Here's how the part is built. I have some questions about the finished solid (model axes, mm). A direction names the side the tool comes from. Give positions to 0.01 mm unless a question says otherwise; leave off trailing zeros. Write each loop counter-clockwise with the first axis right and the second up, starting at its lowest first coordinate (ties: lowest second). Pieces come first, ordered by that corner, then holes. Notation, with made-up numbers: (-32.75, 17) -> (-28.75, 17) arc R35 cw to (-28.75, 49) -> close; hole circle Ø4 at (63.5, -8). An arc over 180 degrees is marked (long way). Use one line per item in the form item = value.
```python
from build123d import *

# Parameters (mm, degrees)
SM_BASE_FLANGE_1_DEPTH = 45
SKETCH_3_R             = 2.1
CUT_EXTRUDE_1_DEPTH    = 105.70434566
SKETCH_4_W             = 35
SKETCH_4_H             = 45
CUT_EXTRUDE_2_DEPTH    = 105.70434566
M3X0_5_1_D             = 2.5
M3X0_5_1_DEPTH         = 7.5
M3X0_5_1_TIP           = 0.751075774
CUT_EXTRUDE_3_DEPTH    = 105.398275848
FILLET_1_R             = 5


# Sheet-metal steps are written as plain solids
with BuildPart() as part:
    # Sketch 1 → 基体-法兰1 (new, symmetric)
    with BuildSketch(Plane(origin=(0, 0, 0), x_dir=(0, 0, -1), z_dir=(1, 0, 0))):
        with BuildLine():
            Line((15, 93), (15, 77.7366))
            ThreePointArc((15, 77.7366), (14.198468417, 75.801531583), (12.2634, 75))
            Line((12.2634, 75), (0.7366, 75))
            ThreePointArc((0.7366, 75), (0.215745145, 74.784254855), (0, 74.2634))
            Line((0, 74.2634), (0, -74.2634))
            ThreePointArc((0, -74.2634), (0.215745145, -74.784254855), (0.7366, -75))
            Line((0.7366, -75), (12.2634, -75))
            ThreePointArc((12.2634, -75), (14.198468417, -75.801531583), (15, -77.7366))
            Line((15, -77.7366), (15, -93))
            Line((15, -93), (13, -93))
            Line((13, -93), (13, -77.7366))
            ThreePointArc((13, -77.7366), (12.784254855, -77.215745145), (12.2634, -77))
            Line((12.2634, -77), (0.7366, -77))
            ThreePointArc((0.7366, -77), (-1.198468417, -76.198468417), (-2, -74.2634))
            Line((-2, -74.2634), (-2, 74.2634))
            ThreePointArc((-2, 74.2634), (-1.198468417, 76.198468417), (0.7366, 77))
            Line((0.7366, 77), (12.2634, 77))
            ThreePointArc((12.2634, 77), (12.784254855, 77.215745145), (13, 77.7366))
            Line((13, 77.7366), (13, 93))
            Line((13, 93), (15, 93))
        make_face()
    extrude(amount=SM_BASE_FLANGE_1_DEPTH, both=True)

    # 草图3 → 切除-拉伸1 (cut, through all)
    with BuildSketch(Plane.XY.offset(2)):
        with Locations((0, 55)):
            Circle(SKETCH_3_R)
        Circle(SKETCH_3_R)
    extrude(amount=-CUT_EXTRUDE_1_DEPTH, mode=Mode.SUBTRACT)

    # 草图4 → 切除-拉伸2 (cut, through all)
    with BuildSketch(Plane.XY.offset(2)):
        with Locations((-27.5, -70.5)):
            Rectangle(SKETCH_4_W, SKETCH_4_H)
    extrude(amount=-CUT_EXTRUDE_2_DEPTH, mode=Mode.SUBTRACT)

    # M3x0.5 螺纹孔1
    with Locations(Plane.XY.offset(2)):
        with Locations((-2.5, -63), (37.5, -63)):
            Hole(M3X0_5_1_D / 2, depth=M3X0_5_1_DEPTH)
            with Locations((0, 0, -(M3X0_5_1_DEPTH + M3X0_5_1_TIP / 2))):  # 118° drill point
                Cone(0, M3X0_5_1_D / 2, M3X0_5_1_TIP, mode=Mode.SUBTRACT)

    # 草图7 → 切除-拉伸3 (cut, through all)
    with BuildSketch(Plane.XY.offset(-13)):
        with BuildLine():
            Line((-30, 88), (-20, 88))
            ThreePointArc((-20, 88), (-17, 85), (-20, 82))
            Line((-20, 82), (-30, 82))
            ThreePointArc((-30, 82), (-33, 85), (-30, 88))
        make_face()
        with BuildLine():
            Line((30, 88), (20, 88))
            ThreePointArc((20, 88), (17, 85), (20, 82))
            Line((20, 82), (30, 82))
            ThreePointArc((30, 82), (33, 85), (30, 88))
        make_face()
        with BuildLine():
            Line((12.5, -82), (22.5, -82))
            ThreePointArc((22.5, -82), (25.5, -85), (22.5, -88))
            Line((22.5, -88), (12.5, -88))
            ThreePointArc((12.5, -88), (9.5, -85), (12.5, -82))
        make_face()
    extrude(amount=-CUT_EXTRUDE_3_DEPTH, mode=Mode.SUBTRACT)

    # 圆角1
    fillet_1_edges = [part.edges().sort_by_distance(p)[0] for p in [
        (-45, 93, -14),
        (45, -93, -14),
        (45, 93, -14),
        (-45, -48, 1),
        (-10, -93, -14),
    ]]
    fillet(fillet_1_edges, radius=FILLET_1_R)


solid = part.part
```
Q1. Which directions (+Z, -Z, +X, -X, +Y, -Y) give clear straight access to the entire face, cutting with the end or side of a thin tool? Please do faces 1 (the face through (18, -89, -13)), 2 (the face through (11, 1, 0)), 3 (the face through (1, 85, -13)), 4 (the face through (-10, -76, -5)).
Result set:
face_1 = +Z, +X, -X, -Y
face_2 = -Z, +X, -X
face_3 = +Z, +X, -X, +Y
face_4 = +Z, -Z, -X, -Y
Q2. Will these pins go through, and if not, where does the flat tip stop? pin 1 Ø6 at (x, z) = (29, -4) entering from +Y; pin 2 Ø10 at (y, z) = (-71.5, -1.5) entering from -X; pin 3 Ø10 at (x, z) = (-16.5, -6.5) entering from -Y.
Result set:
pin_1 = 77
pin_2 = -10
pin_3 = 75
Q3. I want a section at D-D, the plane x = -13.5. Write out the boundary of the cut face in (y, z), and give its area (3 significant figures).
Result set:
outline = (-48, 0) -> (74.26, 0) arc R0.74 cw to (75, -0.74) -> (75, -12.26) arc R2.74 ccw to (77.74, -15) -> (93, -15) -> (93, -13) -> (77.74, -13) arc R0.74 cw to (77, -12.26) -> (77, -0.74) arc R2.74 ccw to (74.26, 2) -> (-48, 2) -> close
area = 309 mm2
Q4. I want a section at A-A, the plane z = -2.5. Write out the boundary of the cut face in (x, y).
Result set:
outline = (-45, 75) -> (45, 75) -> (45, 77) -> (-45, 77) -> close; (-10, -77) -> (45, -77) -> (45, -75) -> (-10, -75) -> close
Q5. If we mould it in two halves opening along Y, with no side actions, what happens to faces 5 (the face through (1, 77, -6)), 6 (the face through (-44, -46, 1)), 7 (the face through (1, 75, -7))? For each: +Y half, -Y half, draft (parallel to the pull), parting line (faces both ways), or undercut.
Result set:
face_5 = +Y half
face_6 = -Y half
face_7 = undercut
Q6. I want a section at C-C, the plane y = 0. Write out the boundary of the cut face in (x, z).
Result set:
outline = (-45, 0) -> (-2.1, 0) -> (-2.1, 2) -> (-45, 2) -> close; (2.1, 0) -> (45, 0) -> (45, 2) -> (2.1, 2) -> close
Q7. If I drill on line 1 along Y through (x, z) = (-6, -10.5); line 2 along Z through (x, y) = (-1, -44); line 3 along Y through (x, z) = (-22, -7.5), over which ranges is the centre line in solid material (lowest first)? Write a range as from..to.
Result set:
line_1 = -77..-75, 75..77
line_2 = 0..2
line_3 = 75..77
Q8. I want a section at B-B, the plane y = 85. Write out the boundary of the cut face in (x, z).
Result set:
outline = (-45, -15) -> (-33, -15) -> (-33, -13) -> (-45, -13) -> close; (-17, -15) -> (17, -15) -> (17, -13) -> (-17, -13) -> close; (33, -15) -> (45, -15) -> (45, -13) -> (33, -13) -> close
